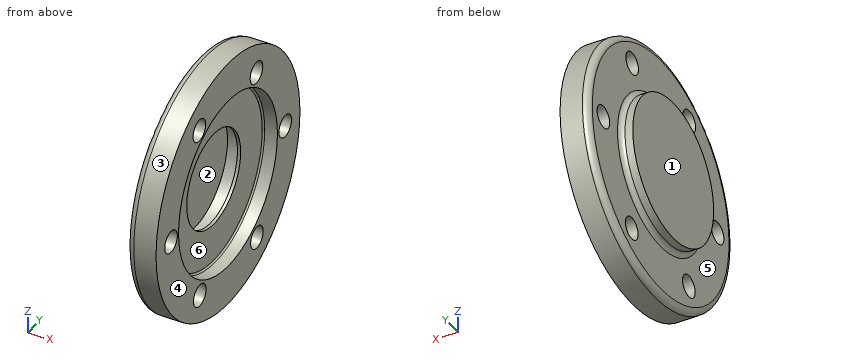
```python
from build123d import *

# Parameters (mm, degrees)
SKETCH2_W              = 14.003667681
SKETCH2_H              = 20
M16X2_0_TAPPED_HOLE1_D = 14
FILLET4_R              = 4
FILLET5_R              = 1


with BuildPart() as part:
    # Sketch1 → Revolve1 (revolve)
    with BuildSketch(Plane(origin=(0, 0, 0), x_dir=(1, 0, 0), z_dir=(0, 1, 0)), mode=Mode.PRIVATE) as revolve1_sk:
        with BuildLine():
            Line((-3.251971734, 30), (-1.251971734, 30))
            Line((-1.251971734, 30), (-1.251971734, 55))
            Line((-1.251971734, 55), (7.748028266, 55))
            Line((7.748028266, 55), (7.748028266, 60))
            Line((7.748028266, 60), (-6.255639415, 60))
            Line((-6.255639415, 60), (-6.255639415, 80))
            Line((-6.255639415, 80), (-10.255639415, 80))
            Line((-10.255639415, 80), (-10.255639415, 48))
            ThreePointArc((-10.255639415, 48), (-11.134319072, 45.878679656), (-13.255639415, 45))
            Line((-13.255639415, 45), (-18.165214358, 45))
            Line((-18.165214358, 45), (-18.165214358, 0))
            Line((-18.165214358, 0), (-13.255639415, 0))
            Line((-13.255639415, 0), (-13.255639415, 36.618791205))
            Line((-13.255639415, 36.618791205), (-3.251971734, 36.618791205))
            Line((-3.251971734, 36.618791205), (-3.251971734, 30))
        make_face()
    revolve(revolve1_sk.sketch.rotate(Axis((0, 0, 0), (1, 0, 0)), 180), axis=Axis((0, 0, 0), (1, 0, 0)))

    # Sketch2 → Revolve2 (revolve)
    with BuildSketch(Plane(origin=(0, 0, 0), x_dir=(1, 0, 0), z_dir=(0, 1, 0)), mode=Mode.PRIVATE) as revolve2_sk:
        with Locations((0.746194426, 70)):
            Rectangle(SKETCH2_W, SKETCH2_H)
    revolve(revolve2_sk.sketch.rotate(Axis((0, 0, 0), (-1, 0, 0)), 180), axis=Axis((0, 0, 0), (-1, 0, 0)))

    # M16x2.0 Tapped Hole1 (through all)
    with Locations(Plane.ZY.offset(10.255639415)):
        with Locations((0, 63.690604398), (54.889736939, 31.690604398), (54.621792488, -31.845302199), (-0.535888903, -63.381208795), (-55.425625842, -31.381208795), (-55.157681391, 32.154697801)):
            Hole(M16X2_0_TAPPED_HOLE1_D / 2)

    # Fillet4
    fillet4_edges = [part.edges().sort_by_distance(p)[0] for p in [
        (-10.255639415, 0, -80),
    ]]
    fillet(fillet4_edges, radius=FILLET4_R)

    # Fillet5
    fillet5_edges = [part.edges().sort_by_distance(p)[0] for p in [
        (-1.251971734, 0, -55),
    ]]
    fillet(fillet5_edges, radius=FILLET5_R)


solid = part.part
```
Work out the finished part from the listing and answer in its coordinate system (mm). Face numbers are marked on the shaded views. A direction names the side the tool comes from. Round coordinates to 2 decimals unless told otherwise and drop trailing zeros. Write each loop counter-clockwise with the first axis right and the second up, starting at its lowest first coordinate (ties: lowest second). Pieces come first, ordered by that corner, then holes. Notation, with made-up numbers: (11, 71) -> (23, 71) arc R11 cw to (23, 89) -> close; hole circle Ø3 at (53, 51). An arc over 180 degrees is marked (long way). Write each question's results on one line, items separated by ' | '.
Q1. Section C-C, the plane z = 0 is taken. Give the number of separate pieces and of enclosed holes in the cut face, then the cut area to 3 significant figures.
Data:
separate pieces: 3 | enclosed holes: 0 | area: 1,240 mm^2
Q2. Which of the six approach directions +Z, -Z, +X, -X, +Y, -Y give full straight-line access (tool end or side, diameter ignored) to the marked faces 4, 5 and 6?
Data:
face 4: +Z, -Z, +X, +Y, -Y | face 5: -X | face 6: +X
Q3. Flat-ended cylindrical pins translate along their axes: P1, Ø22, axis at y = -8.5, z = -14, coming from the +X side; P2, Ø8, axis at x = -0.5, y = 12.5, coming from the -Z side; P3, Ø3, axis at x = -9, y = -37, coming from the -Z side. Find the tip coordinate at first contact, or state that the pin passes through.
Data:
P1: x = -13.26 | P2: z = -79.55 | P3: z = -71.06
Q4. Determine the mould class of the marked faces 1, 2 and 3 for opening direction Z: released by +Z, released by -Z, zero draft, split by the parting line, or undercut.
Data:
face 1: zero draft | face 2: undercut | face 3: split by the parting line
Q5. Section A-A, the plane y = 0 is taken. Write down the section's boundary in (x, z), then the cut area to 3 significant figures.
Data:
outline: (-18.17, -45) -> (-13.26, -45) arc R3 cw to (-10.26, -48) -> (-10.26, -76) arc R4 ccw to (-6.26, -80) -> (7.75, -80) -> (7.75, -55) -> (-0.25, -55) arc R1 cw to (-1.25, -54) -> (-1.25, -30) -> (-3.25, -30) -> (-3.25, -36.62) -> (-13.26, -36.62) -> (-13.26, 36.62) -> (-3.25, 36.62) -> (-3.25, 30) -> (-1.25, 30) -> (-1.25, 54) arc R1 cw to (-0.25, 55) -> (7.75, 55) -> (7.75, 80) -> (-6.26, 80) arc R4 ccw to (-10.26, 76) -> (-10.26, 48) arc R3 cw to (-13.26, 45) -> (-18.17, 45) -> close | area: 1,750 mm^2
Q6. Straight lines are drawn through the part: line 1 along Y through (x, z) = (-2.2, 0); line 2 along Y through (x, z) = (-6, 0); line 3 along Z through (x, y) = (-5.5, -1). For each, find the intervals that lie inside material, in ascending order. Write a range as [from, to].
Data:
line 1: [-80, -70.36], [-56.4, -30], [30, 56.69], [70.69, 80] | line 2: [-80, -70.36], [-56.4, -36.62], [36.62, 56.69], [70.69, 80] | line 3: [-79.99, -36.61], [36.61, 79.99]
Q7. Section B-B, the plane x = 2.25 is taken. Write down the section's boundary in (y, z), then the cut area to 3 significant figures.
Data:
outline: circle Ø160 at (0, 0); hole circle Ø14 at (-63.38, -0.54); hole circle Ø110 at (0, 0); hole circle Ø14 at (-31.85, 54.62); hole circle Ø14 at (-31.38, -55.43); hole circle Ø14 at (31.69, 54.89); hole circle Ø14 at (32.15, -55.16); hole circle Ø14 at (63.69, 0) | area: 9,680 mm^2
Q8. Section D-D, the plane x = -15.75 is taken. Write down the section's boundary in (y, z).
Data:
outline: circle Ø90 at (0, 0)
